Geometry: final body of the model. Coordinates: model frame, mm. Give positions to 0.01 mm unless a question says otherwise; leave off trailing zeros. Order: outer loops, then holes, each group sorted by start corner. A loop starts at its lowest first (then second) coordinate and runs counter-clockwise, first axis right, second up. Notation, with made-up numbers: (-8, -24.5) -> (34, -24.5) arc R4 cw to (34, -18.5) -> close; hole circle Ø6 at (-5.75, 58). An arc over 180 degrees is marked (long way). One line per question, with ' | ' between items.
from build123d import *

# Parameters (mm, degrees)
BOSS_EXTRUDE1_DEPTH = 1.5
SKETCH2_R           = 1.6
CUT_EXTRUDE1_DEPTH  = 3.5


with BuildPart() as part:
    # Sketch1 → Boss-Extrude1 (new body)
    with BuildSketch(Plane.XY):
        Polygon((-586.414001465, 608.080871166), (-828.47776474, 608.080871166), (-828.47776474, 511.530029297), (-586.414001465, 511.530029297), (-586.414001465, 532.14883145), (-600.414001465, 540.231735219), (-600.414001465, 579.379165244), (-586.414001465, 587.462069012), align=None)
    extrude(amount=BOSS_EXTRUDE1_DEPTH)

    # Sketch2 → Cut-Extrude1 (cut)
    with BuildSketch(Plane.XY.offset(1.5)):
        with Locations((-822.47776474, 602.080871166)):
            Circle(SKETCH2_R)
        with Locations((-804.47776474, 602.080871166)):
            Circle(SKETCH2_R)
        with Locations((-822.47776474, 517.530029297)):
            Circle(SKETCH2_R)
        with Locations((-804.47776474, 517.530029297)):
            Circle(SKETCH2_R)
        with Locations((-619.414001465, 602.080871166)):
            Circle(SKETCH2_R)
        with Locations((-592.414001465, 602.080871166)):
            Circle(SKETCH2_R)
        with Locations((-619.414001465, 517.530029297)):
            Circle(SKETCH2_R)
        with Locations((-592.414001465, 517.530029297)):
            Circle(SKETCH2_R)
    extrude(amount=-CUT_EXTRUDE1_DEPTH, mode=Mode.SUBTRACT)


solid = part.part
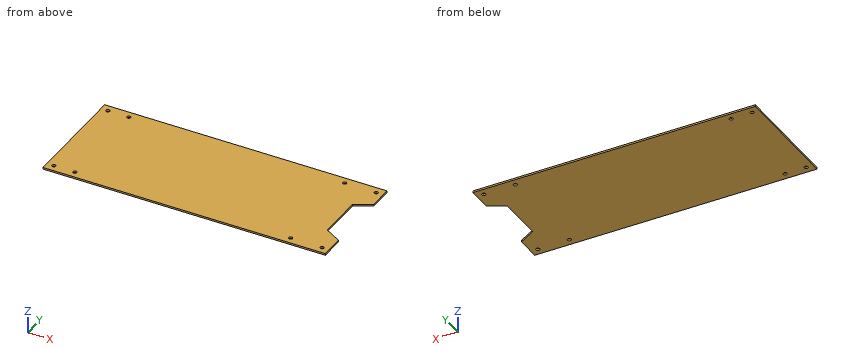
1) Section A-A on z = 1.15. Count the separate pieces of the cut face and the enclosed holes in it, plus the area to 3 significant figures.
Check result:
separate pieces: 1 | enclosed holes: 8 | area: 22,600 mm^2
2) Material intervals for probe 1 along X at (y, z) = (601, 0.3); probe 2 along Y at (x, z) = (-619, 0.8); probe 3 along X at (y, z) = (542.5, 0.9), sorted ascending. Write a range as from..to.
Check result:
probe 1: x = -828.48..-823.66, -821.3..-805.66, -803.3..-620.59, -618.23..-593.59, -591.23..-586.41 | probe 2: y = 511.53..515.98, 519.08..600.54, 603.63..608.08 | probe 3: x = -828.48..-600.41
3) Contact query for flat-ended pins moving along their axis: pin 1 Ø1 at (x, y) = (-687.5, 582) entering from -Z; pin 2 Ø2.5 at (x, y) = (-804.48, 602.08) entering from -Z. Output: stop coordinate, or through.
Check result:
pin 1: stops at z = 0 | pin 2: passes through
4) Section C-C on y = 582. Return loops of the section in (x, z).
Check result:
outline: (-828.48, 0) -> (-595.87, 0) -> (-595.87, 1.5) -> (-828.48, 1.5) -> close
5) Section B-B on y = 547.5. Return loops of the section in (x, z).
Check result:
outline: (-828.48, 0) -> (-600.41, 0) -> (-600.41, 1.5) -> (-828.48, 1.5) -> close
